```python
from build123d import *

# Parameters (mm, degrees)
BOSS_EXTRU_1_DEPTH      = 8
ENL_V_MAT_EXTRU_1_REACH = 183.904
ESQUISSE2_R             = 2.5
BOSS_EXTRU_2_DEPTH      = 2.5
BOSS_EXTRU_2_DEPTH_BACK = 2.5
ESQUISSE4_R             = 2.5


with BuildPart() as part:
    # Esquisse1 → Boss.-Extru.1 (new body)
    with BuildSketch(Plane.XY):
        Polygon((-29, -25), (-29, -10), (-4, -10), (-4, -25), (4, -25), (4, -10), (29, -10), (29, -25), (90, -25), (90, 25), (-90, 25), (-90, -25), align=None)
    extrude(amount=BOSS_EXTRU_1_DEPTH)

    # Enlèv. mat.-Extru.1: up to this face of the body (flat: up to its plane)
    enl_v_mat_extru_1_end = Plane(part.part.faces().sort_by_distance((90, 0, 4))[0])
    # Esquisse2 → Enlèv. mat.-Extru.1 (cut, up to the picked face)
    with BuildSketch(Plane.ZY.offset(90), mode=Mode.PRIVATE) as enl_v_mat_extru_1_sk1:
        with BuildLine():
            add(Edge.make_bspline(
                [(4, -25), (6, -25), (8, -22.5)],
                knots=[0.5, 0.5, 0.5, 1, 1, 1], degree=2))
            Line((4, -25), (8, -25))
            Line((8, -25), (8, -22.5))
        make_face()
    enl_v_mat_extru_1_tool1 = split(extrude(enl_v_mat_extru_1_sk1.sketch, amount=-ENL_V_MAT_EXTRU_1_REACH, mode=Mode.PRIVATE), bisect_by=enl_v_mat_extru_1_end, keep=Keep.BOTH, mode=Mode.PRIVATE)
    # Esquisse2 → Enlèv. mat.-Extru.1 (cut, up to the picked face)
    with BuildSketch(Plane.ZY.offset(90), mode=Mode.PRIVATE) as enl_v_mat_extru_1_sk2:
        with BuildLine():
            add(Edge.make_bspline(
                [(0, -22.5), (2, -25), (4, -25)],
                knots=[0, 0, 0, 0.5, 0.5, 0.5], degree=2))
            Line((0, -22.5), (0, -25))
            Line((0, -25), (4, -25))
        make_face()
    enl_v_mat_extru_1_tool2 = split(extrude(enl_v_mat_extru_1_sk2.sketch, amount=-ENL_V_MAT_EXTRU_1_REACH, mode=Mode.PRIVATE), bisect_by=enl_v_mat_extru_1_end, keep=Keep.BOTH, mode=Mode.PRIVATE)
    # Esquisse2 → Enlèv. mat.-Extru.1 (cut, up to the picked face)
    with BuildSketch(Plane.ZY.offset(90), mode=Mode.PRIVATE) as enl_v_mat_extru_1_sk3:
        with Locations((4, -20)):
            Circle(ESQUISSE2_R)
    enl_v_mat_extru_1_tool3 = split(extrude(enl_v_mat_extru_1_sk3.sketch, amount=-ENL_V_MAT_EXTRU_1_REACH, mode=Mode.PRIVATE), bisect_by=enl_v_mat_extru_1_end, keep=Keep.BOTH, mode=Mode.PRIVATE)
    add(enl_v_mat_extru_1_tool1.solids().sort_by(Axis((-90, -24.25, 7), (1, 0, 0)))[0], mode=Mode.SUBTRACT)
    add(enl_v_mat_extru_1_tool2.solids().sort_by(Axis((-90, -24.25, 1), (1, 0, 0)))[0], mode=Mode.SUBTRACT)
    add(enl_v_mat_extru_1_tool3.solids().sort_by(Axis((-90, -20, 4), (1, 0, 0)))[0], mode=Mode.SUBTRACT)

    # Esquisse4 → Boss.-Extru.2 (add, two sides: drawn at the far end of the back side and taken through both)
    with BuildSketch(Plane(origin=(0, 0, 0), x_dir=(0, 0, -1), z_dir=(1, 0, 0)).offset(-BOSS_EXTRU_2_DEPTH_BACK)):
        with BuildLine():
            Line((5, 4.5), (0, 4.5))
            Line((0, 4.5), (0, -4.5))
            Line((0, -4.5), (5, -4.5))
            ThreePointArc((5, -4.5), (9.5, 0), (5, 4.5))
        make_face()
        with Locations((5, 0)):
            Circle(ESQUISSE4_R, mode=Mode.SUBTRACT)
    extrude(amount=BOSS_EXTRU_2_DEPTH + BOSS_EXTRU_2_DEPTH_BACK)


solid = part.part
```
Work out the finished part from the listing and answer in its coordinate system (mm). A direction names the side the tool comes from. Round coordinates to 2 decimals unless told otherwise and drop trailing zeros. Loops run counter-clockwise (first coordinate to the right, second up) from the corner with the lowest first, then second, coordinate; pieces in that order, holes last.
(1) Each of these flat-tipped pins is pushed along its axis until it touches: P1, Ø8, axis at x = -11.5, y = -1.5, coming from the -Z side; P2, Ø2.5, axis at x = -0.5, z = -2, coming from the -Y side; P3, Ø4.5, axis at y = -1, z = -4, coming from the -X side; P4, Ø4, axis at y = -20, z = 6, coming from the -X side. Where does it stop, or does it pass through?
Computed values:
P1: stops at z = 0
P2: stops at y = -4.5
P3: stops at x = -2.5
P4: stops at x = -90
(2) The mould has two halves that part along Y. Classify faces 6 (the flat face through (0, 4.5, -3)), 7 (the flat face through (0, -4.5, -2)), 8 (the cylindrical face through (-0.035, 0.751, -7.385)), 9 (the cylindrical face through (-0.06, -17.89, 5.34)): pulls with the +Y half, pulls with the -Y half, needs draft (parallel to the pull), parting line crosses it, or undercut.
Computed values:
face 6: pulls with the +Y half
face 7: pulls with the -Y half
face 8: undercut
face 9: undercut
(3) Find the intervals of material crossed by L1, parallel to X at y = -17, z = 4.25; L2, parallel to Y at x = 1.5, z = 4; L3, parallel to Y at x = 1.2, z = -5, in increasing order.
Computed values:
L1: x = -90 to -29, -4 to 4, 29 to 90
L2: y = -25 to -22.5, -17.5 to 25
L3: y = -4.5 to -2.5, 2.5 to 4.5
(4) The part is cut by section A-A, the plane y = 0. Give the vertices of the cut face in (x, z), and give its area (3 significant figures).
Computed values:
outline: (-90, 0) - (-2.5, 0) - (-2.5, -2.5) - (2.5, -2.5) - (2.5, 0) - (90, 0) - (90, 8) - (-90, 8) - close; (-2.5, -9.5) - (2.5, -9.5) - (2.5, -7.5) - (-2.5, -7.5) - close
area: 1,460 mm2
(5) The part is cut by section C-C, the plane x = 22. Give the vertices of the cut face in (y, z).
Computed values:
outline: (-10, 0) - (25, 0) - (25, 8) - (-10, 8) - close
(6) For faces 1 (the flat face through (-1, 2, 8)), 2 (the flat face through (-4, -16, 4)), 3 (the flat face through (2.5, 1.06, -2.57)), 4 (the flat face through (-2.5, 1.06, -2.57)), 5 (the cylindrical face through (0, -0.1, -9.5)), determine the directions among +Z, -Z, +X, -X, +Y, -Y from which every point of the face is accessible in a straight line to the end or side of a thin tool.
Computed values:
face 1: +Z, +X, -X, +Y, -Y
face 2: +Z, -Z, -Y
face 3: -Z, +X, +Y, -Y
face 4: -Z, -X, +Y, -Y
face 5: -Z, +X, -X
(7) The part is cut by section B-B, the plane y = 17.5. Give the vertices of the cut face in (x, z).
Computed values:
outline: (-90, 0) - (90, 0) - (90, 8) - (-90, 8) - close
